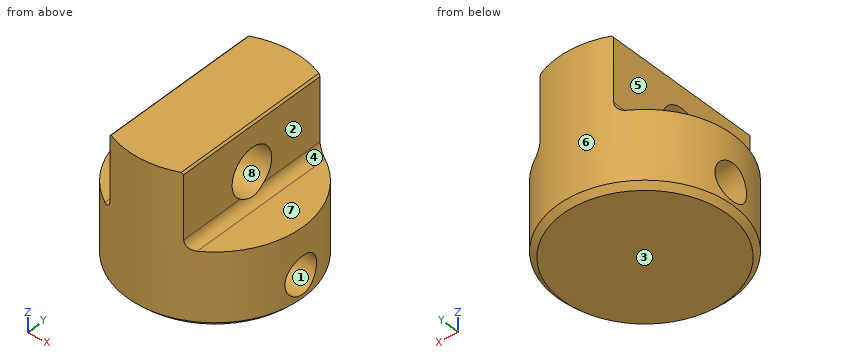
```python
from build123d import *

# Parameters (mm, degrees)
SKETCH_1_R               = 47.5
EXTRUDE_1_DEPTH          = 80
CUT_EXTRUDE_START        = -40
CUT_EXTRUDE_1_DEPTH      = 40
FILLET_1_R               = 5
SKETCH_3_R               = 12.5
CUT_EXTRUDE_2_DEPTH      = 115.945639495
CHAMFER_1_SIZE           = 1
CHAMFER_2_SIZE           = 3
CUT_EXTRUDE_3_DEPTH      = 105.462912246
CUT_EXTRUDE_3_DEPTH_BACK = 105.462912246
SKETCH_4_R               = 10


with BuildPart() as part:
    # Эскиз1 → Бобышка-Вытянуть1 (new body)
    with BuildSketch(Plane.XY):
        Circle(SKETCH_1_R)
    extrude(amount=EXTRUDE_1_DEPTH)

    # Эскиз2 → Вырез-Вытянуть1 (cut)
    with BuildSketch(Plane.XY.offset(80).offset(CUT_EXTRUDE_START)):
        with BuildLine():
            Line((20, -43.084219849), (20, 43.084219849))
            ThreePointArc((20, 43.084219849), (47.5, 0), (20, -43.084219849))
        make_face()
        with BuildLine():
            Line((-20, -43.084219849), (-20, 43.084219849))
            ThreePointArc((-20, 43.084219849), (-47.5, 0), (-20, -43.084219849))
        make_face()
    extrude(amount=CUT_EXTRUDE_1_DEPTH, mode=Mode.SUBTRACT)

    # Скругление1
    fillet_1_edges = [part.edges().sort_by_distance(p)[0] for p in [
        (-20, 0, 40),
        (20, 0, 40),
    ]]
    fillet(fillet_1_edges, radius=FILLET_1_R)

    # Эскиз3 → Вырез-Вытянуть2 (cut, through all)
    with BuildSketch(Plane.ZY.offset(20)):
        with Locations(Location((55, 0, 0), (0, 0, 216.869897646))):
            Circle(SKETCH_3_R)
    extrude(amount=-CUT_EXTRUDE_2_DEPTH, mode=Mode.SUBTRACT)

    # Фаска1
    chamfer_1_edges = [part.edges().sort_by_distance(p)[0] for p in [
        (-20, 0, 80),
        (20, 0, 80),
    ]]
    chamfer(chamfer_1_edges, length=CHAMFER_1_SIZE)

    # Фаска2
    chamfer_2_edges = [part.edges().sort_by_distance(p)[0] for p in [
        (-47.5, 0, 0),
    ]]
    chamfer(chamfer_2_edges, length=CHAMFER_2_SIZE)

    # Эскиз4 → Вырез-Вытянуть3 (cut, two sides: drawn at the far end of the back side and taken through both)
    with BuildSketch(Plane(origin=(0, 0, 0), x_dir=(0, 0, -1), z_dir=(1, 0, 0)).offset(-CUT_EXTRUDE_3_DEPTH_BACK)):
        with Locations((-15, 0)):
            Circle(SKETCH_4_R)
    extrude(amount=CUT_EXTRUDE_3_DEPTH + CUT_EXTRUDE_3_DEPTH_BACK, mode=Mode.SUBTRACT)


solid = part.part
```
Part model, mm, in its own coordinate system. Face numbers are marked on the shaded views. A direction names the side the tool comes from. Coordinates: 2 decimals unless noted, no trailing zeros. Write each loop counter-clockwise with the first axis right and the second up, starting at its lowest first coordinate (ties: lowest second). Pieces come first, ordered by that corner, then holes.
Item 1: Slice it at A-A (y = 0). Write the cut outline in (x, z).
Item 2: Probe line 1 (Z direction, x = -8, y = 0); line 2 (Z direction, x = 4, y = -2.5); line 3 (X direction, y = -19, z = 66). List the from-to ranges inside material, lowest first.
Item 3: Pin check, flat tips, straight feed: pin 1 (2 mm diameter, centred on x = -20.5, y = -12, fed in from +Z); pin 2 (8 mm diameter, centred on x = -31, z = 16, fed in from -Y); pin 3 (12 mm diameter, centred on y = 27, z = 30, fed in from -X); pin 4 (18 mm diameter, centred on y = 0, z = 15, fed in from +X) (3 decimals). Stop position of each tip, or through.
Item 4: Slice it at D-D (z = 30.5). Write the cut outline in (x, y), and give its area (3 significant figures).
Item 5: Slice it at C-C (z = 55). Write the cut outline in (x, y), and give its area (3 significant figures).
Item 6: Slice it at B-B (x = 0). Write the cut outline in (y, z), and give its area (3 significant figures).
Item 7: Which spindle directions (+Z, -Z, +X, -X, +Y, -Y) get a long thin tool onto all of the face, cutting with end or side? Do the marked faces 5, 6, 7 and 8. Say none if no direction does.
Item 8: Mould opens along Z. For the marked faces 1, 2, 3 and 4 say: released by +Z, released by -Z, zero draft, split by the parting line, or undercut.
Results found:
1. outline: (-47.5, 3) - (-44.5, 0) - (44.5, 0) - (47.5, 3) - (47.5, 5) - (-47.5, 5) - close; (-47.5, 25) - (47.5, 25) - (47.5, 40) - (25, 40) arc R5 cw to (20.67, 42.5) - (-20, 42.5) - (-20, 45) arc R5 cw to (-25, 40) - (-47.5, 40) - close; (-20, 67.5) - (20, 67.5) - (20, 79) - (19, 80) - (-19, 80) - (-20, 79) - close
2. line 1: z = 0 to 5, 25 to 42.5, 67.5 to 80
2. line 2: z = 0 to 5.32, 24.68 to 42.75, 67.25 to 80
2. line 3: x = -20 to 20
3. pin 1: stops at z = 79.5
3. pin 2: stops at y = -39.08
3. pin 3: stops at x = -42.61
3. pin 4: passes through
4. outline: circle Ø95 at (0, 0)
4. area: 7,090 mm2
5. outline: (-20, -43.08) arc R47.5 ccw to (20, -43.08) - (20, -12.5) - (-20, -12.5) - close; (-20, 12.5) - (20, 12.5) - (20, 43.08) arc R47.5 ccw to (-20, 43.08) - close
5. area: 2,680 mm2
6. outline: (-47.5, 3) - (-44.5, 0) - (44.5, 0) - (47.5, 3) - (47.5, 80) - (-47.5, 80) - close; hole circle Ø25 at (0, 55); hole circle Ø20 at (0, 15)
6. area: 6,790 mm2
7. face 5: +Z, -X, +Y, -Y
7. face 6: +Z, -Z
7. face 7: +Z, +X, +Y, -Y
7. face 8: +X
8. face 1: undercut
8. face 2: zero draft
8. face 3: released by -Z
8. face 4: released by +Z
